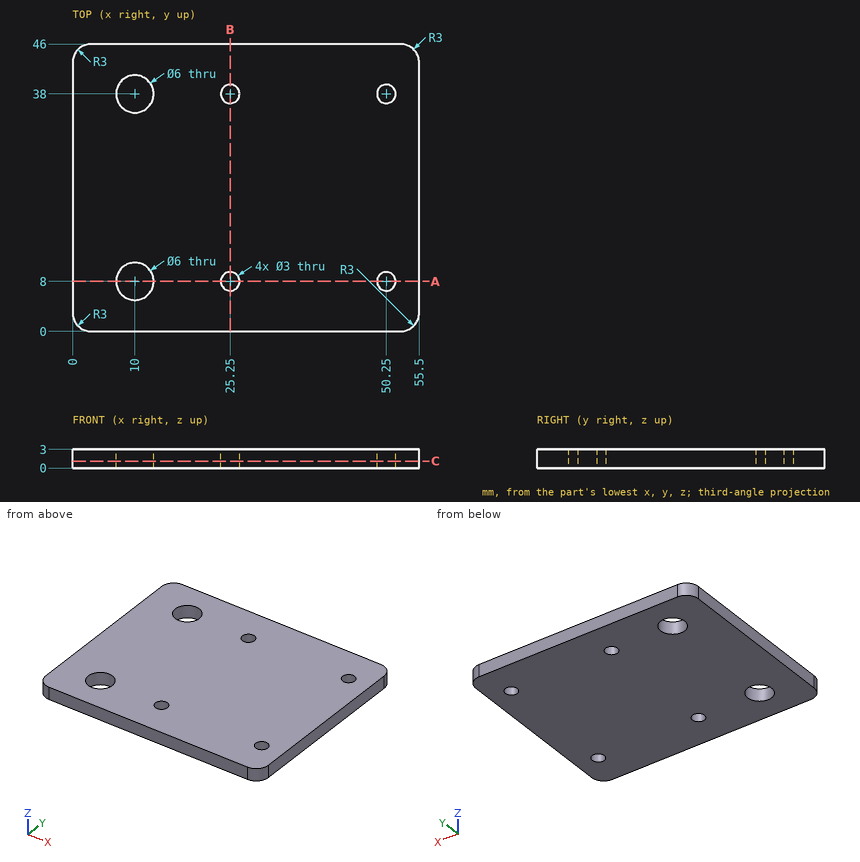
The figure shows three views and two pictorial views of one solid part (mm, origin at its lowest corner). Answer the questions. Round coordinates to 2 decimals unless told otherwise and drop trailing zeros. Write each loop counter-clockwise with the first axis right and the second up, starting at its lowest first coordinate (ties: lowest second). Pieces come first, ordered by that corner, then holes. Notation, with made-up numbers: M -6.5,-16.75 L 2.5,-16.75 A28 ccw 2.5,15.25 Z; hole C -6,-19 d6. An arc over 180 degrees is marked long. Write each question's results on one line, items separated by ' | '. Start each with the question number.
(1) The part is cut by section C-C, the plane z = 1.1. Write down the section's boundary in (x, y).
(2) The part is cut by section B-B, the plane x = 25.25. Write down the section's boundary in (y, z).
(3) The part is cut by section A-A, the plane y = 8. Write down the section's boundary in (x, z).
(4) Find the intervals of material crossed by line 1 (X direction, y = 8, z = 0.85); line 2 (Y direction, x = 25.25, z = 2.4); line 3 (Y direction, x = 10, z = 0.8), in increasing order.
Worked answers:
1) outline: M 0,3 A3 ccw 3,0 L 52.5,0 A3 ccw 55.5,3 L 55.5,43 A3 ccw 52.5,46 L 3,46 A3 ccw 0,43 Z; hole C 10,8 d6; hole C 10,38 d6; hole C 25.25,8 d3; hole C 25.25,38 d3; hole C 50.25,8 d3; hole C 50.25,38 d3
2) outline: M 0,0 L 6.5,0 L 6.5,3 L 0,3 Z; M 9.5,0 L 36.5,0 L 36.5,3 L 9.5,3 Z; M 39.5,0 L 46,0 L 46,3 L 39.5,3 Z
3) outline: M 0,0 L 7,0 L 7,3 L 0,3 Z; M 13,0 L 23.75,0 L 23.75,3 L 13,3 Z; M 26.75,0 L 48.75,0 L 48.75,3 L 26.75,3 Z; M 51.75,0 L 55.5,0 L 55.5,3 L 51.75,3 Z
4) line 1: x = 0 to 7, 13 to 23.75, 26.75 to 48.75, 51.75 to 55.5 | line 2: y = 0 to 6.5, 9.5 to 36.5, 39.5 to 46 | line 3: y = 0 to 5, 11 to 35, 41 to 46
